Part model, mm, in its own coordinate system. Face numbers are marked on the shaded views. A direction names the side the tool comes from. Give positions to 0.01 mm unless a question says otherwise; leave off trailing zeros. Loops run counter-clockwise (first coordinate to the right, second up) from the corner with the lowest first, then second, coordinate; pieces in that order, holes last. Notation, with made-up numbers: (60.25, -14) -> (64.25, -14) arc R16 cw to (64.25, -1) -> close; hole circle Ø10 at (56.5, 23.25). An arc over 180 degrees is marked (long way). One line per question, with ' | ' between items.
```python
from build123d import *

# Parameters (mm, degrees)
EXTRUDE_1_DEPTH = 0.3
SKETCH_2_R      = 3.5
EXTRUDE_2_DEPTH = 12


with BuildPart() as part:
    # 草图1 → 凸台-拉伸1 (new body)
    with BuildSketch(Plane(origin=(0, 0, 0), x_dir=(1, 0, 0), z_dir=(0, 1, 0))):
        with BuildLine():
            Line((-8, 0), (-8, 8))
            Line((-8, 8), (8, 8))
            Line((8, 8), (8, 0))
            ThreePointArc((8, 0), (6.164414003, -5.099019514), (1.5, -7.858116823))
            Line((1.5, -7.858116823), (1.5, -15.858116823))
            Line((1.5, -15.858116823), (-1.5, -15.858116823))
            Line((-1.5, -15.858116823), (-1.5, -7.858116823))
            ThreePointArc((-1.5, -7.858116823), (-6.164414003, -5.099019514), (-8, 0))
        make_face()
    extrude(amount=EXTRUDE_1_DEPTH)

    # 草图2 → 凸台-拉伸2 (add)
    with BuildSketch(Plane(origin=(0, 0.3, 0), x_dir=(1, 0, 0), z_dir=(0, 1, 0))):
        with Locations(Location((0, 0, 0), (0, 0, 270))):
            Circle(SKETCH_2_R)
    extrude(amount=EXTRUDE_2_DEPTH)


solid = part.part
```
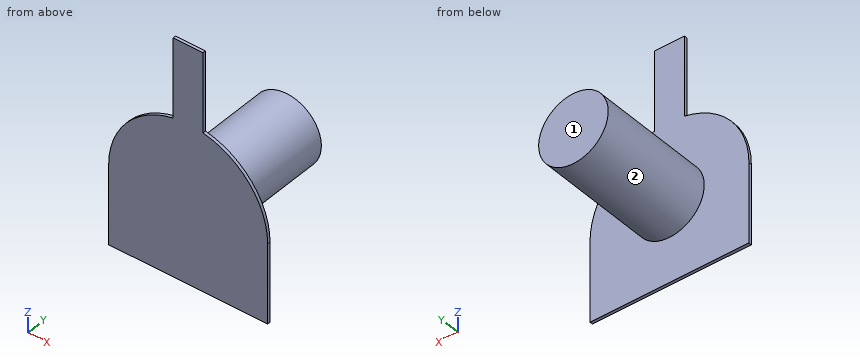
1) Saw through at D-D (x = 2.75). Give the cut face in (y, z), and give its area (3 significant figures).
Found:
outline: (0, -8) -> (0.3, -8) -> (0.3, -2.17) -> (12.3, -2.17) -> (12.3, 2.17) -> (0.3, 2.17) -> (0.3, 7.51) -> (0, 7.51) -> close | area: 56.6 mm2
2) Saw through at C-C (z = -6.25). Give the cut face in (x, y), and give its area (3 significant figures).
Found:
outline: (-8, 0) -> (8, 0) -> (8, 0.3) -> (-8, 0.3) -> close | area: 4.80 mm2
3) Drill centre lines: line 1 (Y direction, x = 3.75, z = -5.25); line 2 (X direction, y = 5.5, z = 2.75); line 3 (X direction, y = 11, z = 3). Where is each one in solid material? Low to high.
Found:
line 1: 0 to 0.3 | line 2: -2.17 to 2.17 | line 3: -1.8 to 1.8
4) Pin check, flat tips, straight feed: P1, Ø1, axis at y = 1.5, z = -1.5, coming from the -X side; P2, Ø3, axis at x = 6, y = 10.5, coming from the -Z side; P3, Ø3, axis at x = -2, z = 6.5, coming from the +Y side. Stop position of each tip, or through.
Found:
P1: x = -3.35 | P2: through | P3: y = 0.3
5) Tool access for the marked faces 1 and 2: list every direction of +Z, -Z, +X, -X, +Y, -Y with a clear straight run to the whole face (end or side of a thin tool).
Found:
face 1: +Z, -Z, +X, -X, +Y | face 2: +Y
6) Saw through at A-A (x = 0). Give the cut face in (y, z).
Found:
outline: (0, -8) -> (0.3, -8) -> (0.3, -3.5) -> (12.3, -3.5) -> (12.3, 3.5) -> (0.3, 3.5) -> (0.3, 15.86) -> (0, 15.86) -> close
7) Saw through at B-B (y = 9.75). Give the cut face in (x, z), and give its area (3 significant figures).
Found:
outline: circle Ø7 at (0, 0) | area: 38.5 mm2
